from build123d import *

# Parameters (mm, degrees)
SKETCH_R     = 11.5
PAD_DEPTH    = 15
SKETCH001_R  = 12.5
PAD001_DEPTH = 3
FILLET_R     = 1


with BuildPart() as part:
    # Sketch → Pad (new body)
    with BuildSketch(Plane.XY):
        Circle(SKETCH_R)
    extrude(amount=PAD_DEPTH)

    # Sketch001 (on DatumPlane) → Pad001 (join)
    with BuildSketch(Plane.XY.offset(15)):
        Circle(SKETCH001_R)
    extrude(amount=PAD001_DEPTH)

    # Fillet
    fillet_edges = [part.edges().sort_by_distance(p)[0] for p in [
        (-12.5, 0, 18),
    ]]
    fillet(fillet_edges, radius=FILLET_R)


solid = part.part
Work out the finished part from the listing and answer in its coordinate system (mm). A direction names the side the tool comes from. Give positions to 0.01 mm unless a question says otherwise; leave off trailing zeros. Order: outer loops, then holes, each group sorted by start corner. A loop starts at its lowest first (then second) coordinate and runs counter-clockwise, first axis right, second up. Notation, with made-up numbers: (33, 85) -> (68, 85) arc R14 cw to (68, 99) -> close; hole circle Ø2 at (-20.5, 51.25). An arc over 180 degrees is marked (long way). One line per item, written item: value.
Item 1: Find section C-C, the plane z = 15.75. Give the vertices of the cut face in (x, y).
Answer sheet:
outline: circle Ø25 at (0, 0)
Item 2: A tool of negligible diameter and unlimited length cuts with its end or side. For faces 1 (the flat face through (0, 0, 0)), 2 (the cylindrical face through (-1.5, 11.4, 7.4)), from which of +Z, -Z, +X, -X, +Y, -Y can it reach the whole face along a straight path? Write none if from no direction.
Answer sheet:
face 1: -Z, +X, -X, +Y, -Y
face 2: -Z
Item 3: Flat-ended cylindrical pins translate along their axes: P1, Ø4, axis at x = -8.5, z = 13, coming from the +Y side; P2, Ø5, axis at y = -7, z = 8.5, coming from the -X side; P3, Ø3, axis at x = 7, z = 10, coming from the -Y side. Find the tip coordinate at first contact, or state that the pin passes through.
Answer sheet:
P1: y = 9.49
P2: x = -10.58
P3: y = -10.1
Item 4: Find section A-A, the plane y = 0. Give the vertices of the cut face in (x, z).
Answer sheet:
outline: (-12.5, 15) -> (-11.5, 15) -> (-11.5, 0) -> (11.5, 0) -> (11.5, 15) -> (12.5, 15) -> (12.5, 17) arc R1 ccw to (11.5, 18) -> (-11.5, 18) arc R1 ccw to (-12.5, 17) -> close
Item 5: Straight lines are drawn through the part: probe 1 along X at (y, z) = (7.25, 12.25); probe 2 along Y at (x, z) = (11, 16.75); probe 3 along X at (y, z) = (-9.5, 5). For each, find the intervals that lie inside material, in ascending order.
Answer sheet:
probe 1: -8.93 to 8.93
probe 2: -5.94 to 5.94
probe 3: -6.48 to 6.48
